Verification items for this drawing (mm, ordinates from the low corner). Coordinates: 2 decimals unless noted, no trailing zeros. Write each loop counter-clockwise with the first axis right and the second up, starting at its lowest first coordinate (ties: lowest second). Pieces come first, ordered by that corner, then holes.
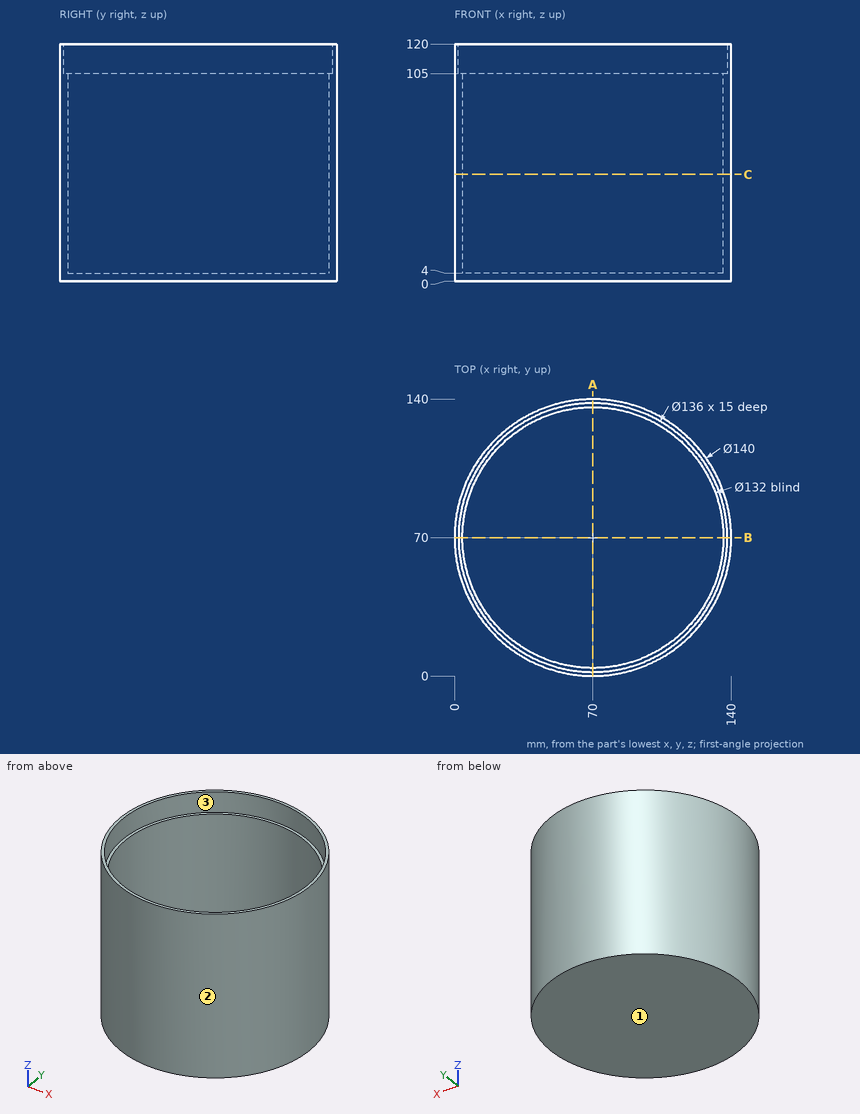
1. Sectioned sample at A-A, the plane x = 70. Record the boundary of the cut face in (y, z).
Computed values:
outline: (0, 0) - (140, 0) - (140, 120) - (138, 120) - (138, 105) - (136, 105) - (136, 4) - (4, 4) - (4, 105) - (2, 105) - (2, 120) - (0, 120) - close
2. Gauge pin test, flat ends, axial feed: pin 1 Ø10 at (x, y) = (124.5, 101.5) entering from +Z; pin 2 Ø8 at (y, z) = (24, 51.5) entering from +X; pin 3 Ø1 at (y, z) = (55.5, 95) entering from -X. Record the tip position at first contact, or that the pin passes through.
Computed values:
pin 1: stops at z = 105
pin 2: stops at x = 126
pin 3: stops at x = 1.41
3. Draft check along Y on the marked faces 1, 2 and 3. Enter one of: released by +Y, released by -Y, zero draft, split by the parting line, or undercut.
Computed values:
face 1: zero draft
face 2: split by the parting line
face 3: undercut
4. Sectioned sample at C-C, the plane z = 54. Record the boundary of the cut face in (x, y), and give its area (3 significant figures).
Computed values:
outline: circle Ø140 at (70, 70); hole circle Ø132 at (70, 70)
area: 1,710 mm2
5. Thickness scan on line 1 along Y through (x, z) = (70, 73); line 2 along Z through (x, y) = (130.5, 74); line 3 along X through (y, z) = (64.5, 75.5). Record the ranges inside material, lowest first.
Computed values:
line 1: y = 0 to 4, 136 to 140
line 2: z = 0 to 4
line 3: x = 0.22 to 4.23, 135.77 to 139.78
